Check sheet for the modelled part. Datum: model origin and axes. Units: mm. A direction names the side the tool comes from. Round coordinates to 2 decimals unless told otherwise and drop trailing zeros. Loops run counter-clockwise (first coordinate to the right, second up) from the corner with the lowest first, then second, coordinate; pieces in that order, holes last. Notation, with made-up numbers: (47.25, 83.25) -> (84.25, 83.25) arc R22 cw to (84.25, 100.25) -> close; hole circle Ø9 at (29.5, 61). An arc over 180 degrees is marked (long way). Return JSON: item names as keys, results as strings.
from build123d import *

# Parameters (mm, degrees)
EXTRUDE_1_DEPTH = 16
EXTRUDE_START   = 2
EXTRUDE_2_DEPTH = 2


with BuildPart() as part:
    # 草图2 → 凸台-拉伸1 (new body)
    with BuildSketch(Plane.XY):
        with BuildLine():
            Line((-48.762908832, 54.887448723), (-26.762908832, 54.887448723))
            Line((-26.762908832, 54.887448723), (-26.762908832, 41.887448723))
            Line((-26.762908832, 41.887448723), (-32.402449776, 41.887448723))
            Line((-32.402449776, 41.887448723), (-36.699855568, 9.854978503))
            ThreePointArc((-36.699855568, 9.854978503), (-37.727531794, -4.542394165), (-33.311876123, -18.284389767))
            Line((-33.311876123, -18.284389767), (-24.708766903, -24.263803058))
            Line((-24.708766903, -24.263803058), (-28.738435498, -27.878766712))
            Line((-28.738435498, -27.878766712), (-30.734862705, -29.630628791))
            ThreePointArc((-30.734862705, -29.630628791), (-33.621940029, -30.923968409), (-36.736058642, -30.367005118))
            Line((-36.736058642, -30.367005118), (-39.496815638, -28.94354271))
            ThreePointArc((-39.496815638, -28.94354271), (-41.356176764, -27.633440822), (-42.78903224, -25.866942609))
            ThreePointArc((-42.78903224, -25.866942609), (-49.053565639, -9.682339493), (-49.408404924, 7.668736722))
            Line((-49.408404924, 7.668736722), (-44.097278331, 41.887448723))
            Line((-44.097278331, 41.887448723), (-48.762908832, 41.887448723))
            Line((-48.762908832, 41.887448723), (-48.762908832, 54.887448723))
        make_face()
        with BuildLine():
            Line((-30.065808903, -26.382705226), (-32.053997966, -28.127338346))
            ThreePointArc((-32.053997966, -28.127338346), (-33.865522987, -28.938856991), (-35.819507294, -28.589384904))
            Line((-35.819507294, -28.589384904), (-38.580264289, -27.165922497))
            ThreePointArc((-38.580264289, -27.165922497), (-39.990623798, -26.172186191), (-41.077470951, -24.832264904))
            ThreePointArc((-41.077470951, -24.832264904), (-47.091423014, -9.295045913), (-47.432068727, 7.361987253))
            Line((-47.432068727, 7.361987253), (-41.762908832, 43.887448723))
            Line((-41.762908832, 43.887448723), (-46.762908832, 43.887448723))
            Line((-46.762908832, 43.887448723), (-46.762908832, 52.887448723))
            Line((-46.762908832, 52.887448723), (-28.762908832, 52.887448723))
            Line((-28.762908832, 52.887448723), (-28.762908832, 43.887448723))
            Line((-28.762908832, 43.887448723), (-34.152052224, 43.887448723))
            Line((-34.152052224, 43.887448723), (-38.66514404, 10.247274583))
            ThreePointArc((-38.66514404, 10.247274583), (-39.67581399, -5.082301073), (-34.833871303, -19.66218223))
            Line((-34.833871303, -19.66218223), (-27.926153972, -24.463248422))
            Line((-27.926153972, -24.463248422), (-30.065808903, -26.382705226))
        make_face(mode=Mode.SUBTRACT)
    extrude(amount=EXTRUDE_1_DEPTH)

    # 草图3 → 凸台-拉伸2 (add)
    with BuildSketch(Plane(origin=(0, 0, 0), x_dir=(-1, 0, 0), z_dir=(0, 0, -1)).offset(EXTRUDE_START)):
        with BuildLine():
            Line((24.708766903, -24.263803058), (33.311876123, -18.284389767))
            ThreePointArc((33.311876123, -18.284389767), (37.727531794, -4.542394165), (36.699855568, 9.854978503))
            Line((36.699855568, 9.854978503), (32.402449776, 41.887448723))
            Line((32.402449776, 41.887448723), (26.762908832, 41.887448723))
            Line((26.762908832, 41.887448723), (26.762908832, 54.887448723))
            Line((26.762908832, 54.887448723), (48.762908832, 54.887448723))
            Line((48.762908832, 54.887448723), (48.762908832, 41.887448723))
            Line((48.762908832, 41.887448723), (44.097278331, 41.887448723))
            Line((44.097278331, 41.887448723), (49.408404924, 7.668736722))
            ThreePointArc((49.408404924, 7.668736722), (49.053565639, -9.682339493), (42.78903224, -25.866942609))
            ThreePointArc((42.78903224, -25.866942609), (41.356176764, -27.633440822), (39.496815638, -28.94354271))
            Line((39.496815638, -28.94354271), (36.736058642, -30.367005118))
            ThreePointArc((36.736058642, -30.367005118), (33.621940029, -30.923968409), (30.734862705, -29.630628791))
            Line((30.734862705, -29.630628791), (28.738435498, -27.878766712))
            Line((28.738435498, -27.878766712), (24.708766903, -24.263803058))
        make_face()
    extrude(amount=-EXTRUDE_2_DEPTH)


solid = part.part
Q1. Material ranges on line 1 (Y direction, x = -29.5, z = 9.5); line 2 (X direction, y = 46.5, z = 12.75); line 3 (X direction, y = 0.5, z = -0.25), recorded low to high.
Results list:
{"line 1": "-28.55 to -25.88, -23.37 to -20.93, 41.89 to 43.89, 52.89 to 54.89", "line 2": "-48.76 to -46.76, -28.76 to -26.76", "line 3": "-50 to -38"}
Q2. Draft check along X on faces 4 (the flat face through (-38, 54.887, 7)), 5 (the cylindrical face through (-49.1, -9.44, 6.87)), 6 (the flat face through (-28.763, 48, 8)). Enter one of: released by +X, released by -X, zero draft, split by the parting line, or undercut.
Results list:
{"face 4": "zero draft", "face 5": "released by -X", "face 6": "undercut"}
Q3. Section check A-A (y = 46). Record the boundary of the cut face in (x, z), then the cut area to 3 significant figures.
Results list:
{"outline": "(-48.76, -2) -> (-26.76, -2) -> (-26.76, 16) -> (-28.76, 16) -> (-28.76, 0) -> (-46.76, 0) -> (-46.76, 16) -> (-48.76, 16) -> close", "area": "108 mm^2"}
Q4. Go/stop test with flat-tipped pins: pin 1 (10 mm diameter, centred on y = 48, z = 7, fed in from -X); pin 2 (8 mm diameter, centred on x = -41, z = 8, fed in from -Y); pin 3 (10 mm diameter, centred on x = -33.5, z = 1, fed in from -Y); pin 4 (10.5 mm diameter, centred on y = 51, z = 10.5, fed in from +X). Record where each tip stops, or that it passes through.
Results list:
{"pin 1": "x = -48.76", "pin 2": "y = -30.23", "pin 3": "y = -30.96", "pin 4": "x = -26.76"}
Q5. Section check C-C (y = -6.5). Record the boundary of the cut face in (x, z), then the cut area to 3 significant figures.
Results list:
{"outline": "(-49.58, -2) -> (-37.44, -2) -> (-37.44, 16) -> (-39.47, 16) -> (-39.47, 0) -> (-47.56, 0) -> (-47.56, 16) -> (-49.58, 16) -> close", "area": "89.0 mm^2"}
Q6. Tool access check on faces 1 (the flat face through (-31, -27.2, 7.9)), 2 (the flat face through (-30, 41.887, 7)), 3 (the flat face through (-26.763, 48, 7)). Record the directions out of +Z, -Z, +X, -X, +Y, -Y that give a thin tool (end or side, any length) a straight path to the whole face; none if there is none.
Results list:
{"face 1": "+Z", "face 2": "+Z, -Z, +X", "face 3": "+Z, -Z, +X, +Y"}
